Design review of the part built by this model. Coordinates are the model's own, in mm. Face numbers are marked on the shaded views. A direction names the side the tool comes from. Coordinates: 2 decimals unless noted, no trailing zeros. Loops run counter-clockwise (first coordinate to the right, second up) from the corner with the lowest first, then second, coordinate; pieces in that order, holes last. Notation, with made-up numbers: M -14.5,16.25 L 17.5,16.25 A28 ccw 17.5,50.25 Z; hole C 39,-11.5 d3. An arc over 180 degrees is marked long. One line per item, written item: value.
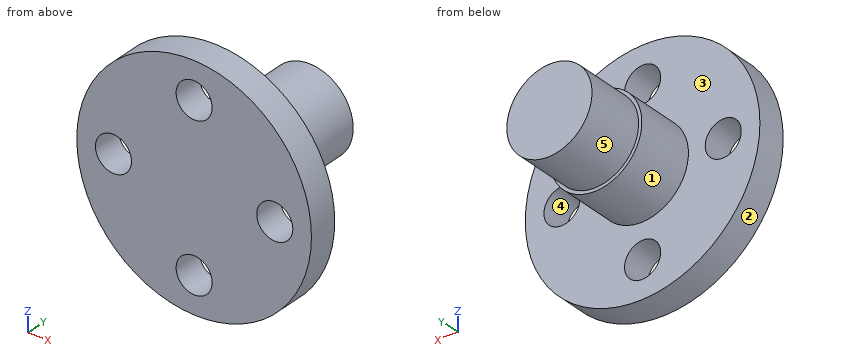
```python
from build123d import *

# Parameters (mm, degrees)
F0_R     = 4.6125
F1_DEPTH = 6.35
F2_R     = 4.9625
F3_DEPTH = 6.35
F4_R     = 12.7
F4_R_2   = 1.9526
F5_DEPTH = 3.175


# Not quite as in the source:
# - a length typed as a fraction of an inch, garbled in the dataset ("3 / 203.2 mm" for 3/8 in), is restored


with BuildPart() as f1:
    # F0 (on Front) → F1 (new body)
    with BuildSketch(Plane.XZ):
        Circle(F0_R)
    extrude(amount=F1_DEPTH)

    # F2 (on face) → F3 (join)
    with BuildSketch(Plane.XZ.offset(6.35)):
        Circle(F2_R)
    extrude(amount=F3_DEPTH)

    # F4 (on face) → F5 (join)
    with BuildSketch(Plane.XZ.offset(12.7)):
        Circle(F4_R)
        with Locations((0, -8.73125)):
            Circle(F4_R_2, mode=Mode.SUBTRACT)
        with Locations((-8.73125, 0)):
            Circle(F4_R_2, mode=Mode.SUBTRACT)
        with Locations((8.73125, 0)):
            Circle(F4_R_2, mode=Mode.SUBTRACT)
        with Locations((0, 8.73125)):
            Circle(F4_R_2, mode=Mode.SUBTRACT)
    extrude(amount=F5_DEPTH)


solid = f1.part
```
(1) Tool access review of the marked faces 1 and 2: name each direction out of +Z, -Z, +X, -X, +Y, -Y from which nothing blocks a thin tool from reaching the whole face with its end or side.
Reply:
face 1: +Y
face 2: +Y, -Y
(2) We need section A-A on x = 0. State how many separate pieces and enclosed holes the cut face has, then the cut area to 3 significant figures.
Reply:
separate pieces: 3
enclosed holes: 0
area: 177 mm2
(3) Mouldability with a two-part tool opening along X and no side actions: class the marked faces 3, 4 and 5 as released by +X, released by -X, zero draft, split by the parting line, or undercut.
Reply:
face 3: zero draft
face 4: undercut
face 5: split by the parting line
(4) Insertion check: pin 1 (4.5 mm diameter, centred on x = 0, z = 8.73, fed in from +Y); pin 2 (3.5 mm diameter, centred on x = 0, z = -8.73, fed in from -Y); pin 3 (1 mm diameter, centred on y = -3, z = 0.5, fed in from +X). Each pin has a flat end and moves straight along its axis. Give the tip position at first contact, or say it passes through.
Reply:
pin 1: stops at y = -12.7
pin 2: passes through
pin 3: stops at x = 4.61
(5) To check wall thickness, follow line 1 along Z through (x, y) = (0, -14.2); line 2 along Y through (x, z) = (-5.25, 0.25) (3 decimals); line 3 along Z through (x, y) = (7.5, -14). State the ranges of each line that lie inside material, in increasing order. Write a range as [from, to].
Reply:
line 1: z = [-12.7, -10.68], [-6.78, 6.78], [10.68, 12.7]
line 2: y = [-15.875, -12.7]
line 3: z = [-10.25, -1.52], [1.52, 10.25]
(6) We need section D-D on x = 8. State the section outline as (y, z) points (1 decimal), then the cut area to 3 significant figures.
Reply:
outline: M -15.9,-9.9 L -12.7,-9.9 L -12.7,-1.8 L -15.9,-1.8 Z; M -15.9,1.8 L -12.7,1.8 L -12.7,9.9 L -15.9,9.9 Z
area: 51.1 mm2
(7) We need section C-C on z = -10. State the section outline as (x, y) points (3 decimals), then the cut area to 3 significant figures.
Reply:
outline: M -7.829,-15.875 L -1.484,-15.875 L -1.484,-12.7 L -7.829,-12.7 Z; M 1.484,-15.875 L 7.829,-15.875 L 7.829,-12.7 L 1.484,-12.7 Z
area: 40.3 mm2
